Here's the drawing with two shaded views (mm, measured from the low corner). I have some questions. A direction names the side the tool comes from. Coordinates: 2 decimals unless noted, no trailing zeros. Loops run counter-clockwise (first coordinate to the right, second up) from the corner with the lowest first, then second, coordinate; pieces in that order, holes last. Notation, with made-up numbers: M 20,26.25 L 65,26.25 A23 ccw 65,64.25 Z; hole C 1,80.5 d7. An arc over 180 degrees is marked long. Return JSON: item names as keys, results as strings. Group by question number.
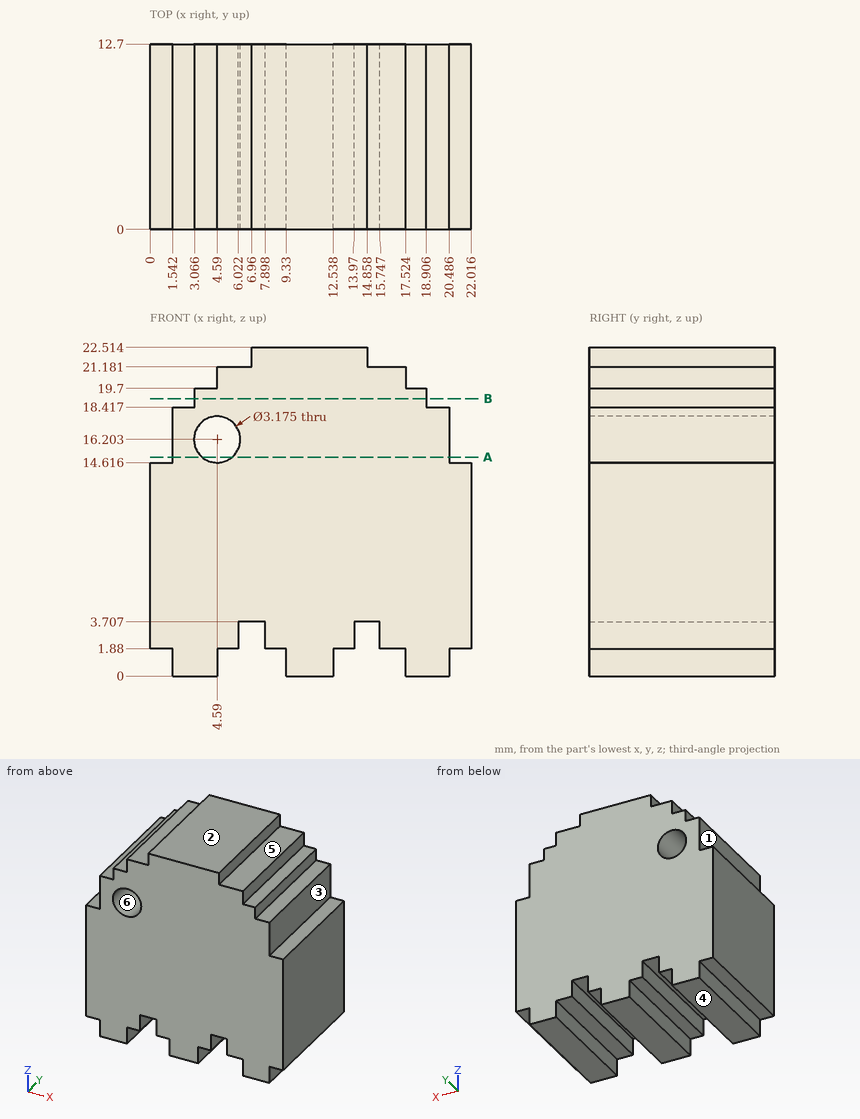
1) For pin 1 (1.5 mm diameter, centred on y = 9, z = 0.5, fed in from +X); pin 2 (2 mm diameter, centred on x = 16.5, y = 7.5, fed in from +Z); pin 3 (1.7 mm diameter, centred on x = 20, y = 4, fed in from +Z), each with a flat end and sliding along its axis, tell me the tip position at first contact or that it passes through.
2) If we mould it in two halves opening along Z, with no side actions, what happens to the marked faces 3, 4, 5 and 6? For each: +Z half, -Z half, draft (parallel to the pull), parting line (faces both ways), or undercut.
3) Suppose I cut it at A-A, the plane z = 15. List the corners of the cut face in (x, y) for me (1 decimal), then the cut area to 3 significant figures.
4) Suppose I cut it at B-B, the plane z = 19. List the corners of the cut face in (x, y) for me, then the cut area to 3 significant figures.
5) If I drill on line 1 (X direction, y = 4.75, z = 1.75) (1 decimal); line 2 (Z direction, x = 16.5, y = 4); line 3 (Z direction, x = 7.25, y = 4.5), over which ranges is the centre line in solid material (lowest first)? Write a range as from..to.
6) For the marked faces 1 and 2, which set-ups out of +Z, -Z, +X, -X, +Y, -Y let a thin tool reach every point of the face, with its end or its side?
Returned:
{
 "1": {"pin 1": "stops at x = 20.49", "pin 2": "stops at z = 21.18", "pin 3": "stops at z = 18.42"},
 "2": {"face 3": "draft", "face 4": "-Z half", "face 5": "+Z half", "face 6": "undercut"},
 "3": {"outline": "M 1.5,0 L 3.6,0 L 3.6,12.7 L 1.5,12.7 Z; M 5.6,0 L 20.5,0 L 20.5,12.7 L 5.6,12.7 Z", "area": "214 mm²"},
 "4": {"outline": "M 3.07,0 L 18.91,0 L 18.91,12.7 L 3.07,12.7 Z", "area": "201 mm²"},
 "5": {"line 1": "x = 1.5..4.6, 9.3..12.5, 17.5..20.5", "line 2": "z = 1.88..21.18", "line 3": "z = 3.71..22.51"},
 "6": {"face 1": "+Z, -X, +Y, -Y", "face 2": "+Z, +X, -X, +Y, -Y"}
}
